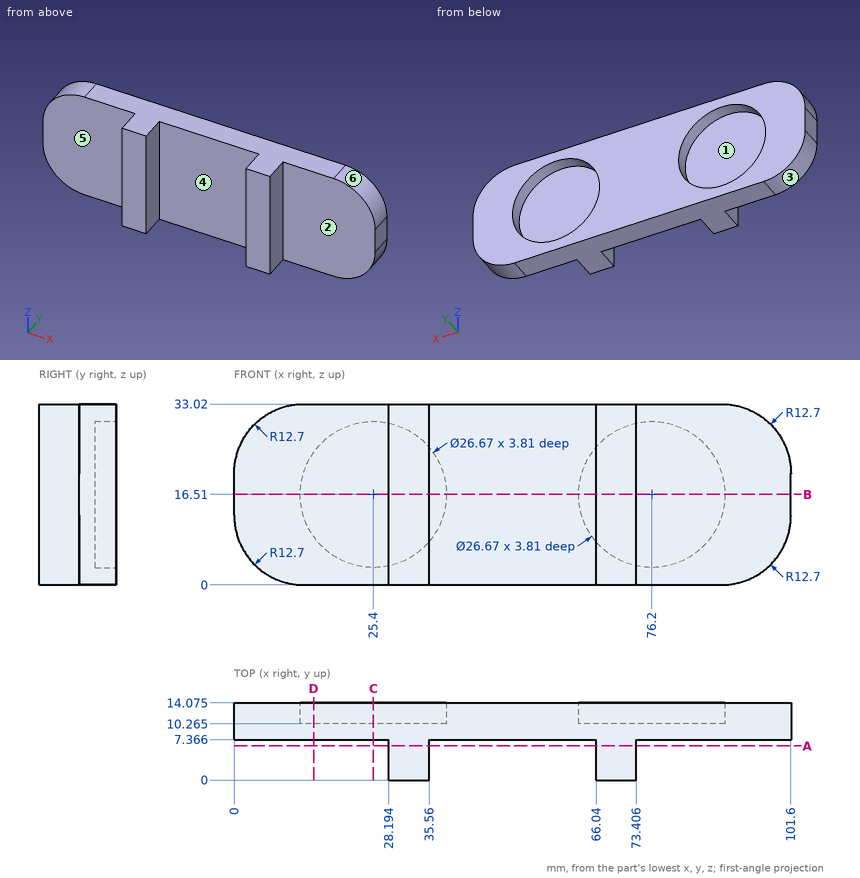
Drawing for the job (mm, zero at the part's lowest x, y, z). A direction names the side the tool comes from. Give positions to 0.01 mm unless a question says otherwise; leave off trailing zeros. Loops run counter-clockwise (first coordinate to the right, second up) from the corner with the lowest first, then second, coordinate; pieces in that order, holes last.
(1) Pull direction X, two halves, no side cores. Call the marked faces 4, 5 and 6: pulls with the +X half, pulls with the -X half, needs draft (parallel to the pull), parting line crosses it, or undercut.
Return value:
face 4: undercut
face 5: needs draft
face 6: pulls with the +X half
(2) 3-axis set-ups, long thin cutter, end or side, ignore diameter. For the marked faces 1, 2 and 3: which of +Z, -Z, +X, -X, +Y, -Y reach the whole face in a straight line?
Return value:
face 1: +Y
face 2: +Z, -Z, +X, -Y
face 3: -Z, -X, +Y, -Y
(3) Band-saw the part on D-D (x = 14.5). Write the cut outline in (y, z) (1 decimal).
Return value:
outline: (7.4, 0) - (14.1, 0) - (14.1, 8.8) - (10.3, 8.8) - (10.3, 24.2) - (14.1, 24.2) - (14.1, 33) - (7.4, 33) - close
(4) Drill centre lines: line 1 along X through (y, z) = (6.5, 15.5); line 2 along Z through (x, y) = (76.2, 11.9) (1 decimal); line 3 along X through (y, z) = (10.75, 5.5) (1 decimal). Where is each one in solid material? Low to high.
Return value:
line 1: x = 28.19 to 35.56, 66.04 to 73.41
line 2: z = 0 to 3.2, 29.8 to 33
line 3: x = 2.2 to 17.9, 32.9 to 68.7, 83.7 to 99.4
(5) Band-saw the part on C-C (x = 25.4). Write the cut outline in (y, z) (1 decimal), and give its area (3 significant figures).
Return value:
outline: (7.4, 0) - (14.1, 0) - (14.1, 3.2) - (10.3, 3.2) - (10.3, 29.8) - (14.1, 29.8) - (14.1, 33) - (7.4, 33) - close
area: 120 mm2
(6) Band-saw the part on A-A (y = 6.25). Write the cut outline in (x, z).
Return value:
outline: (28.19, 0) - (35.56, 0) - (35.56, 33.02) - (28.19, 33.02) - close; (66.04, 0) - (73.41, 0) - (73.41, 33.02) - (66.04, 33.02) - close
(7) Band-saw the part on B-B (z = 16.51). Write the cut outline in (x, y) (1 decimal), and give its area (3 significant figures).
Return value:
outline: (0, 7.4) - (28.2, 7.4) - (28.2, 0) - (35.6, 0) - (35.6, 7.4) - (66, 7.4) - (66, 0) - (73.4, 0) - (73.4, 7.4) - (101.6, 7.4) - (101.6, 14.1) - (89.5, 14.1) - (89.5, 10.3) - (62.9, 10.3) - (62.9, 14.1) - (38.7, 14.1) - (38.7, 10.3) - (12.1, 10.3) - (12.1, 14.1) - (0, 14.1) - close
area: 587 mm2
(8) Pin check, flat tips, straight feed: pin 1 (1.5 mm diameter, centred on x = 23.5, z = 22.5, fed in from -Y); pin 2 (3 mm diameter, centred on y = 4, z = 26, fed in from +X); pin 3 (2 mm diameter, centred on y = 4, z = 19.5, fed in from -X). Stop position of each tip, or through.
Return value:
pin 1: stops at y = 7.37
pin 2: stops at x = 73.41
pin 3: stops at x = 28.19
